```python
from build123d import *

# Parameters (mm, degrees)
F1_DEPTH = 25
F2_R     = 4.5
F3_DEPTH = 7.001


# Not quite as in the source:
# - a pattern or mirror of a feature is missing from the dataset's text; its kind, count and spacing are read off the source's solid


with BuildPart() as f1:
    # F0 (on Front) → F1 (new body, symmetric)
    with BuildSketch(Plane.XZ):
        with BuildLine():
            ThreePointArc((-28.2506073348, 0), (0, 28.2506073348), (28.2506073348, 0))
            Line((28.2506073348, 0), (65.5786693096, 0))
            Line((65.5786693096, 0), (65.5786693096, 7))
            Line((65.5786693096, 7), (34.5485935672, 7))
            ThreePointArc((34.5485935672, 7), (0, 35.2506073348), (-34.5485935672, 7))
            Line((-34.5485935672, 7), (-62.9629269242, 7))
            Line((-62.9629269242, 7), (-62.9629269242, 0))
            Line((-62.9629269242, 0), (-28.2506073348, 0))
        make_face()
    extrude(amount=F1_DEPTH, both=True)

    # F2 (on face) → F3 (cut, through all)
    with BuildSketch(Plane.XY.offset(7)):
        with Locations((-48.7557602457, -12.5)):
            Circle(F2_R)
        with Locations((-48.7557602457, 12.5)):
            Circle(F2_R)
    f3 = extrude(amount=-F3_DEPTH, mode=Mode.SUBTRACT)

    # F3_copies: F3 across plane
    add(f3.mirror(Plane(origin=(0, 0, 0), x_dir=(0, 0, 1), z_dir=(1, 0, 0))), mode=Mode.SUBTRACT)


solid = f1.part
```
Geometry check sheet. Reference: the model listing, model coordinates, mm. A direction names the side the tool comes from. Give positions to 0.01 mm unless a question says otherwise; leave off trailing zeros. Write each loop counter-clockwise with the first axis right and the second up, starting at its lowest first coordinate (ties: lowest second). Pieces come first, ordered by that corner, then holes.
1) Gauge pin test, flat ends, axial feed: pin 1 (4 mm diameter, centred on y = -12.5, z = 20, fed in from +X); pin 2 (4 mm diameter, centred on y = -1.5, z = 25, fed in from +X); pin 3 (12 mm diameter, centred on y = 12.5, z = 31, fed in from -X); pin 4 (5.5 mm diameter, centred on x = -48.76, y = -12.5, fed in from -Z). Record the tip position at first contact, or that the pin passes through.
2) Access from +Z, -Z, +X, -X, +Y, -Y to the whole of each face (thin tool, end or side, straight path). Record for faces 4 (the flat face through (-49, 0, 7)), 5 (the cylindrical face through (0.677, -0.35, 35.244)), 6 (the flat face through (50, 0, 7)).
3) Section check D-D, the plane x = 0. Record the boundary of the cut face in (y, z).
4) Release check for a two-part mould opening along Y. For faces 1 (the flat face through (6, 25, 28)), 2 (the cylindrical face through (44.464, 13.852, 3.549)), 3 (the flat face through (-46, 0, 0)) record: pulls with the +Y half, pulls with the -Y half, needs draft (parallel to the pull), parting line crosses it, or undercut.
5) Section check C-C, the plane y = -5. Record the boundary of the cut face in (x, z), and give its area (3 significant figures).
6) Material ranges on L1, parallel to X at y = 12, z = 1; L2, parallel to Y at x = 52, z = 6; L3, parallel to Z at x = 37, y = -9.5, recorded low to high.
7) Section check B-B, the plane z = 26.5. Record the boundary of the cut face in (x, y), and give its area (3 significant figures).
8) Section check A-A, the plane y = -12.5. Record the boundary of the cut face in (x, z).
Computed:
1. pin 1: stops at x = 30.31
1. pin 2: stops at x = 26.71
1. pin 3: stops at x = -24.85
1. pin 4: passes through
2. face 4: +Z, -X, +Y, -Y
2. face 5: +Z, +Y, -Y
2. face 6: +Z, +X, +Y, -Y
3. outline: (-25, 28.25) - (25, 28.25) - (25, 35.25) - (-25, 35.25) - close
4. face 1: pulls with the +Y half
4. face 2: undercut
4. face 3: needs draft
5. outline: (-62.96, 0) - (-28.25, 0) arc R28.25 cw to (28.25, 0) - (65.58, 0) - (65.58, 7) - (34.55, 7) arc R35.25 ccw to (-34.55, 7) - (-62.96, 7) - close
5. area: 1,110 mm2
6. L1: x = -62.96 to -53.23, -44.28 to -28.23, 28.23 to 44.28, 53.23 to 65.58
6. L2: y = -25 to -15.62, -9.38 to 9.38, 15.62 to 25
6. L3: z = 0 to 7
7. outline: (-23.25, -25) - (-9.79, -25) - (-9.79, 25) - (-23.25, 25) - close; (9.79, -25) - (23.25, -25) - (23.25, 25) - (9.79, 25) - close
7. area: 1,350 mm2
8. outline: (-62.96, 0) - (-53.26, 0) - (-53.26, 7) - (-62.96, 7) - close; (-44.26, 0) - (-28.25, 0) arc R28.25 cw to (28.25, 0) - (44.26, 0) - (44.26, 7) - (34.55, 7) arc R35.25 ccw to (-34.55, 7) - (-44.26, 7) - close; (53.26, 0) - (65.58, 0) - (65.58, 7) - (53.26, 7) - close
